```python
from build123d import *

# Parameters (mm, degrees)
F0_W     = 83
F0_H     = 7.6
F0_W_2   = 79.5
F0_H_2   = 2.6
F1_DEPTH = 7
F2_W     = 83
F2_H     = 7.6
F2_W_2   = 79.5
F2_H_2   = 2.6
F3_DEPTH = 3.2
F4_W     = 3
F4_H     = 2
F4_W_2   = 5.4
F4_H_2   = 5.4
F4_H_3   = 2.8
F5_DEPTH = 6


with BuildPart() as f1:
    # F0 (on Front) → F1 (new body)
    with BuildSketch(Plane.XZ):
        Rectangle(F0_W, F0_H)
        Rectangle(F0_W_2, F0_H_2, mode=Mode.SUBTRACT)
    extrude(amount=F1_DEPTH)

    # F2 (on face) → F3 (join)
    with BuildSketch(Plane.XZ.offset(7)):
        Rectangle(F2_W, F2_H)
        Rectangle(F2_W_2, F2_H_2, mode=Mode.SUBTRACT)
        Rectangle(F2_W_2, F2_H_2)
    extrude(amount=F3_DEPTH)

    # F4 (on face) → F5 (join)
    with BuildSketch(Plane.XY.offset(3.8)):
        with Locations((-40, -9.2)):
            Rectangle(F4_W, F4_H)
        with Locations((-35.8, -9.2)):
            Rectangle(F4_W_2, F4_H)
        with Locations((-40, -5.5)):
            Rectangle(F4_W, F4_H_2)
        with Locations((-31.6, -9.2)):
            Rectangle(F4_W, F4_H)
        with Locations((-40, -1.4)):
            Rectangle(F4_W, F4_H_3)
        with Locations((-31.6, -5.5)):
            Rectangle(F4_W, F4_H_2)
        with Locations((-35.8, -1.4)):
            Rectangle(F4_W_2, F4_H_3)
        with Locations((-23.2, -9.2)):
            Rectangle(F4_W, F4_H)
        with Locations((-31.6, -1.4)):
            Rectangle(F4_W, F4_H_3)
        with Locations((-19, -9.2)):
            Rectangle(F4_W_2, F4_H)
        with Locations((-23.2, -5.5)):
            Rectangle(F4_W, F4_H_2)
        with Locations((-14.8, -9.2)):
            Rectangle(F4_W, F4_H)
        with Locations((-23.2, -1.4)):
            Rectangle(F4_W, F4_H_3)
        with Locations((-14.8, -5.5)):
            Rectangle(F4_W, F4_H_2)
        with Locations((-19, -1.4)):
            Rectangle(F4_W_2, F4_H_3)
        with Locations((-14.8, -1.4)):
            Rectangle(F4_W, F4_H_3)
        with Locations((14.8, -9.2)):
            Rectangle(F4_W, F4_H)
        with Locations((19, -9.2)):
            Rectangle(F4_W_2, F4_H)
        with Locations((14.8, -5.5)):
            Rectangle(F4_W, F4_H_2)
        with Locations((23.2, -9.2)):
            Rectangle(F4_W, F4_H)
        with Locations((14.8, -1.4)):
            Rectangle(F4_W, F4_H_3)
        with Locations((23.2, -5.5)):
            Rectangle(F4_W, F4_H_2)
        with Locations((19, -1.4)):
            Rectangle(F4_W_2, F4_H_3)
        with Locations((31.6, -9.2)):
            Rectangle(F4_W, F4_H)
        with Locations((23.2, -1.4)):
            Rectangle(F4_W, F4_H_3)
        with Locations((35.8, -9.2)):
            Rectangle(F4_W_2, F4_H)
        with Locations((31.6, -5.5)):
            Rectangle(F4_W, F4_H_2)
        with Locations((40, -9.2)):
            Rectangle(F4_W, F4_H)
        with Locations((31.6, -1.4)):
            Rectangle(F4_W, F4_H_3)
        with Locations((40, -5.5)):
            Rectangle(F4_W, F4_H_2)
        with Locations((35.8, -1.4)):
            Rectangle(F4_W_2, F4_H_3)
        with Locations((40, -1.4)):
            Rectangle(F4_W, F4_H_3)
    extrude(amount=F5_DEPTH)


solid = f1.part
```
Here's how the part is built. I have some questions about the finished solid (model axes, mm). A direction names the side the tool comes from. Coordinates: 2 decimals unless noted, no trailing zeros. Order: outer loops, then holes, each group sorted by start corner. A loop starts at its lowest first (then second) coordinate and runs counter-clockwise, first axis right, second up. Notation, with made-up numbers: (-16, -15.75) - (20, -15.75) arc R18 cw to (20, 17.25) - close; hole circle Ø7 at (63.5, 76.25). An arc over 180 degrees is marked (long way). One line per question, with ' | ' between items. Start each with the question number.
1. If we section it at A-A (z = 6.5): Give the number of separate pieces and of enclosed holes in the cut face, and give its area (3 significant figures).
2. Which directions (+Z, -Z, +X, -X, +Y, -Y) give clear straight access to the entire face, cutting with the end or side of a thin tool? Please do faces 1 (the flat face through (41.5, -5, 3)), 2 (the flat face through (19, -2.8, 7)), 3 (the flat face through (30.1, -5, 7)).
3. I'm going to push a flat-ended pin straight in: pin 1 Ø1.6 at (x, y) = (-19.5, -5) entering from +Z. Where does the tip first touch, or does it pass through?
4. If we mould it in two halves opening along Z, with no side actions, what happens to faces 4 (the flat face through (-1, -7, 0)), 5 (the flat face through (-19, -2, 9.8)), 6 (the flat face through (36, -2.8, 7)), 7 (the flat face through (-39.75, -3, 0))? For each: released by +Z, released by -Z, zero draft, split by the parting line, or undercut.
5. If we section it at C-C (x = -19): Write out the boundary of the cut face in (y, z), and give its area (3 significant figures).
6. If we section it at D-D (z = 0.5): Write out the boundary of the cut face in (x, y), and give its area (3 significant figures).
7. Please list where these lines run through material, in increasing order: line 1 along X through (y, z) = (-1, 4); line 2 along Z through (x, y) = (-5, -4.5); line 3 along X through (y, z) = (-4, 1.25). Write a range as [from, to].
8. If we section it at B-B (y = -9): Write out the boundary of the cut face in (x, z).
Model answer:
1) separate pieces: 4 | enclosed holes: 4 | area: 348 mm²
2) face 1: +Z, -Z, +X, +Y, -Y | face 2: +Z | face 3: +Z, +Y, -Y
3) pin 1: stops at z = 3.8
4) face 4: undercut | face 5: released by +Z | face 6: zero draft | face 7: undercut
5) outline: (-10.2, -3.8) - (0, -3.8) - (0, -1.3) - (-7, -1.3) - (-7, 1.3) - (0, 1.3) - (0, 9.8) - (-2.8, 9.8) - (-2.8, 3.8) - (-8.2, 3.8) - (-8.2, 9.8) - (-10.2, 9.8) - close | area: 88.1 mm²
6) outline: (-41.5, -10.2) - (41.5, -10.2) - (41.5, 0) - (39.75, 0) - (39.75, -7) - (-39.75, -7) - (-39.75, 0) - (-41.5, 0) - close | area: 290 mm²
7) line 1: x = [-41.5, -30.1], [-24.7, -13.3], [13.3, 24.7], [30.1, 41.5] | line 2: z = [-3.8, -1.3], [1.3, 3.8] | line 3: x = [-41.5, -39.75], [39.75, 41.5]
8) outline: (-41.5, -3.8) - (41.5, -3.8) - (41.5, 9.8) - (30.1, 9.8) - (30.1, 3.8) - (24.7, 3.8) - (24.7, 9.8) - (13.3, 9.8) - (13.3, 3.8) - (-13.3, 3.8) - (-13.3, 9.8) - (-24.7, 9.8) - (-24.7, 3.8) - (-30.1, 3.8) - (-30.1, 9.8) - (-41.5, 9.8) - close
